```python
from build123d import *

# Parameters (mm, degrees)
SKETCH_1_R          = 4.5
EXTRUDE_1_DEPTH     = 5
SKETCH_2_R          = 4.25
EXTRUDE_2_DEPTH     = 5
SKETCH_3_R          = 2.25
CUT_EXTRUDE_1_DEPTH = 18
CUT_EXTRUDE_2_REACH = 91.037
SKETCH_4_W          = 30
SKETCH_4_H          = 2


with BuildPart() as part:
    # 스케치1 → 보스-돌출1 (new body)
    with BuildSketch(Plane.XY):
        with BuildLine():
            Line((5, 5.590169944), (75, 5.590169944))
            ThreePointArc((75, 5.590169944), (87.5, 0), (75, -5.590169944))
            Line((75, -5.590169944), (5, -5.590169944))
            ThreePointArc((5, -5.590169944), (-7.5, 0), (5, 5.590169944))
        make_face()
        Circle(SKETCH_1_R, mode=Mode.SUBTRACT)
    extrude(amount=EXTRUDE_1_DEPTH)

    # 스케치2 → 보스-돌출2 (add)
    with BuildSketch(Plane.XY.offset(5)):
        with Locations((80, 0)):
            Circle(SKETCH_2_R)
    extrude(amount=EXTRUDE_2_DEPTH)

    # 스케치3 → 컷-돌출1 (cut)
    with BuildSketch(Plane.XY.offset(10)):
        with Locations((80, 0)):
            Circle(SKETCH_3_R)
    extrude(amount=-CUT_EXTRUDE_1_DEPTH, mode=Mode.SUBTRACT)

    # 스케치4 → 컷-돌출2 (cut, up to next)
    with BuildSketch(Plane(origin=(0, 5.590169944, 0), x_dir=(1, 0, 0), z_dir=(0, 1, 0)), mode=Mode.PRIVATE) as cut_extrude_2_sk1:
        with Locations((27.5, -1)):
            Rectangle(SKETCH_4_W, SKETCH_4_H)
    cut_extrude_2_tool1 = extrude(cut_extrude_2_sk1.sketch, amount=-CUT_EXTRUDE_2_REACH, mode=Mode.PRIVATE) & part.part
    add(cut_extrude_2_tool1.solids().sort_by_distance((27.5, 5.59017, 1))[0], mode=Mode.SUBTRACT)


solid = part.part
```
Check sheet for the modelled part. Datum: model origin and axes. Units: mm. A direction names the side the tool comes from. Round coordinates to 2 decimals unless told otherwise and drop trailing zeros. Loops run counter-clockwise (first coordinate to the right, second up) from the corner with the lowest first, then second, coordinate; pieces in that order, holes last. Notation, with made-up numbers: (12.5, -6) - (61.5, -6) arc R13 ccw to (61.5, 5) - close; hole circle Ø5 at (33, -17). An arc over 180 degrees is marked (long way). Write item = value, one per line. Start each with the question number.
Q1. Section check D-D (x = 41.5). Record the boundary of the cut face in (y, z).
Q2. Section check A-A (y = 0). Record the boundary of the cut face in (x, z), plus the area to 4 significant figures.
Q3. Access from +Z, -Z, +X, -X, +Y, -Y to the whole of each face (thin tool, end or side, straight path). Record for faces 4 (the face through (12.5, 0, 1)), 5 (the face through (40, 5.59, 3)), 6 (the face through (65, 0, 0)), 7 (the face through (40, -5.59, 3)).
Q4. Section check B-B (y = 6.5). Record the boundary of the cut face in (x, z), plus the area to 3 significant figures.
Q5. Thickness scan on L1, parallel to X at y = -3, z = 1.25; L2, parallel to Y at x = 80, z = 4.75; L3, parallel to Z at x = 60.5, y = -5. Record the ranges inside material, lowest first.
Q6. Depth check by flat-ended pin: P1, Ø5.5, axis at x = 43.5, z = 2.5, coming from the -Y side; P2, Ø1, axis at y = -1.5, z = 1, coming from the -X side; P3, Ø4, axis at x = 13, z = 6.5, coming from the +Y side; P4, Ø2.5, axis at x = 80, y = 0, coming from the +Z side. Enter the tip coordinate at first touch or a pass-through.
Q7. Release check for a two-part mould opening along X. For faces 1 (the face through (-0.59, 4.46, 2.46)), 2 (the face through (82, -2, 10)), 3 (the face through (84.054, 1.277, 7.465)) record: pulls with the +X half, pulls with the -X half, needs draft (parallel to the pull), parting line crosses it, or undercut.
Q8. Section check C-C (z = 7.5). Record the boundary of the cut face in (x, y).
Derived:
q1.outline = (-5.59, 2) - (5.59, 2) - (5.59, 5) - (-5.59, 5) - close
q2.outline = (-7.5, 0) - (-4.5, 0) - (-4.5, 5) - (-7.5, 5) - close; (4.5, 0) - (12.5, 0) - (12.5, 2) - (42.5, 2) - (42.5, 0) - (77.75, 0) - (77.75, 10) - (75.75, 10) - (75.75, 5) - (4.5, 5) - close; (82.25, 0) - (87.5, 0) - (87.5, 5) - (84.25, 5) - (84.25, 10) - (82.25, 10) - close
q2.area = 367.5 mm^2
q3.face_4 = -Z, +Y, -Y
q3.face_5 = +Z, -Z, +Y
q3.face_6 = -Z, +X, -X, +Y, -Y
q3.face_7 = +Z, -Z, -Y
q4.outline = (-3.74, 0) - (3.74, 0) - (3.74, 5) - (-3.74, 5) - close; (76.26, 0) - (83.74, 0) - (83.74, 5) - (76.26, 5) - close
q4.area = 74.8 mm^2
q5.L1 = -6.87 to -3.35, 3.35 to 12.5, 42.5 to 86.87
q5.L2 = -7.5 to -2.25, 2.25 to 7.5
q5.L3 = 0 to 5
q6.P1 = -5.59
q6.P2 = -7.43
q6.P3 = 5.59
q6.P4 = through
q7.face_1 = undercut
q7.face_2 = needs draft
q7.face_3 = parting line crosses it
q8.outline = circle Ø8.5 at (80, 0); hole circle Ø4.5 at (80, 0)
